The listing builds one solid part. Answer for the finished solid, in the listing's coordinates (mm). Give positions to 0.01 mm unless a question says otherwise; leave off trailing zeros. Order: outer loops, then holes, each group sorted by start corner. A loop starts at its lowest first (then second) coordinate and runs counter-clockwise, first axis right, second up. Notation, with made-up numbers: (47, 52) - (94, 52) arc R10 ccw to (94, 58) - close; hole circle Ø10 at (73, 55). An arc over 180 degrees is marked (long way). Answer as a JSON object with one key per item and string values. Group by question number.
Q1. A cutting plane is placed at D-D, the plane x = -3.55. Give the vertices of the cut face in (y, z).
Q2. Consider line 1 (Z direction, x = -2.55, y = 0.55); line 2 (X direction, y = 0.25, z = -32.25); line 3 (Z direction, x = -2.7, y = 2.2). Determine where each line is inside the solid, lowest interval first.
Q3. A cutting plane is placed at C-C, the plane y = 0.8. Give the vertices of the cut face in (x, z), and give its area (3 significant figures).
Q4. A cutting plane is placed at B-B, the plane x = -1.9. Give the vertices of the cut face in (y, z).
Q5. The mould has two halves that part along Z. Classify faces 1 (the face through (-3, 1, -34.8)), 2 (the face through (0, 1, -20)), 3 (the face through (-2.151, 1.183, -6.097)): released by +Z, released by -Z, zero draft, split by the parting line, or undercut.
Q6. A cutting plane is placed at A-A, the plane z = -32.2. Give the vertices of the cut face in (x, y), and give its area (3 significant figures).
Q7. Given pin 1 (3 mm diameter, centred on x = -2, z = -10, fed in from -Y); pin 2 (3 mm diameter, centred on x = -2.53, z = -7.81, fed in from -Y), each flat-ended and moving along its own axis, determine where each tip first touches the part or whether it passes through.
Autodesk Inventor part; units mm, degrees
ref_plane "YZ Plane" through (0, 0, 0) normal (1, 0, 0) x (0, 1, 0)
ref_plane "XZ Plane" through (0, 0, 0) normal (0, 1, 0) x (-1, 0, 0)
ref_plane "XY Plane" through (0, 0, 0) normal (0, 0, 1) x (1, 0, 0)
sketch "Эскиз2" plane through (0, 0, 0) normal (0, 1, 0) x (-1, 0, 0)
  circle A0 centre (2.5304, -32.2) radius 1.75
  line L0 (0, -30.0054) -> (5, -30.0054)
  line L1 (0, -34.8) -> (0, -30.0054)
  line L2 (5, -34.8) -> (0, -34.8)
  line L3 (5, -30.0054) -> (5, -34.8)
  line L4 (0, -16) -> (5, -16)
  line L5 (0, -24.0054) -> (0, -16)
  line L6 (5, -24.0054) -> (0, -24.0054)
  line L7 (5, -16) -> (5, -24.0054)
  circle A1 centre (2.5304, -7.8054) radius 1.75
  line L8 (5, -10) -> (0, -10)
  line L9 (5, -5) -> (5, -10)
  line L10 (0, -5) -> (5, -5)
  line L11 (0, -10) -> (0, -5)
  line L12 (5, -5) -> (0, -5)
  line L13 (0, -5) -> (0, -34.8)
  line L14 (0, -34.8) -> (5, -34.8)
  line L15 (5, -34.8) -> (5, -5)
  point P0 (0, 0)
  point P1 (5, 0)
extrude "Выдавливание2" add sketch "Эскиз2" along normal blind 2.4
properties part number "КВ33.044.406 - Прижим ремня" material "Пластик АБС"
Reply:
{
 "1": {"outline": "(0, -34.8) - (2.4, -34.8) - (2.4, -33.62) - (0, -33.62) - close; (0, -30.78) - (2.4, -30.78) - (2.4, -9.23) - (0, -9.23) - close; (0, -6.38) - (2.4, -6.38) - (2.4, -5) - (0, -5) - close"},
 "2": {"line 1": "z = -34.8 to -33.95, -30.45 to -9.56, -6.06 to -5", "line 2": "x = -5 to -4.28, -0.78 to 0", "line 3": "z = -34.8 to -33.94, -30.46 to -9.55, -6.06 to -5"},
 "3": {"outline": "(-5, -34.8) - (0, -34.8) - (0, -5) - (-5, -5) - close; hole circle Ø3.5 at (-2.53, -32.2); hole circle Ø3.5 at (-2.53, -7.81)", "area": "130 mm^2"},
 "4": {"outline": "(0, -34.8) - (2.4, -34.8) - (2.4, -33.83) - (0, -33.83) - close; (0, -30.57) - (2.4, -30.57) - (2.4, -9.44) - (0, -9.44) - close; (0, -6.17) - (2.4, -6.17) - (2.4, -5) - (0, -5) - close"},
 "5": {"face 1": "released by -Z", "face 2": "zero draft", "face 3": "undercut"},
 "6": {"outline": "(-5, 0) - (-4.28, 0) - (-4.28, 2.4) - (-5, 2.4) - close; (-0.78, 0) - (0, 0) - (0, 2.4) - (-0.78, 2.4) - close", "area": "3.60 mm^2"},
 "7": {"pin 1": "stops at y = 0", "pin 2": "passes through"}
}
